Here's how the part is built. I have some questions about the finished solid (model axes, mm). A direction names the side the tool comes from. Round coordinates to 2 decimals unless told otherwise and drop trailing zeros. Write each loop counter-clockwise with the first axis right and the second up, starting at its lowest first coordinate (ties: lowest second). Pieces come first, ordered by that corner, then holes. Notation, with made-up numbers: (42.5, -10.75) - (80.5, -10.75) arc R23 ccw to (80.5, 28.25) - close; hole circle Ø11 at (66.25, 56.5). An arc over 180 degrees is marked (long way). Write item = value, one per line. Start each with the question number.
Item 1: Which directions (+Z, -Z, +X, -X, +Y, -Y) give clear straight access to the entire face, cutting with the end or side of a thin tool? Please do faces 4 (the face through (-26.398, -13, -27)), 5 (the face through (39.733, -13, 32)), 6 (the face through (39.733, -13, -32)), 7 (the face through (8, -25.4, -28)).
Item 2: If I drill on line 1 along Z through (x, y) = (-10, -7.5); line 2 along X through (y, z) = (-26, -14.5); line 3 along Z through (x, y) = (12, 2.5) (3 decimals), over which ranges is the centre line in solid material (lowest first)? Write a range as [from, to].
Item 3: If we section it at B-B (y = -20): Please give me the cut outline in (x, z) (3 decimals).
Item 4: Thinking about a two-plate mould opening in Z: for faces 1 (the face through (7, -33.02, 0)), 2 (the face through (-1, -13, 46.809)), 3 (the face through (-17.83, -12.88, -35.8)), which applies, pulls with the +Z half, pulls with the -Z half, needs draft (parallel to the pull), parting line crosses it, or undercut?
Item 5: For P1, Ø21, axis at y = -18.5, z = 25.5, coming from the -X side; P2, Ø1, axis at x = 27.5, z = 22.5, coming from the -Y side; P3, Ø20.5, axis at y = -18, z = 32, coming from the +X side, each with a flat end and sliding along its axis, tell me the tip position at first contact or that it passes through.
Item 6: If we section it at D-D (x = 29): Please give me the cut outline in (y, z) (3 decimals), and give its area (3 significant figures).
Item 7: If we section it at C-C (z = -33): Please give me the cut outline in (x, y).
Item 8: If we section it at A-A (x = 2.5): Please give me the cut outline in (y, z) (3 decimals).
```python
from build123d import *

# Parameters (mm, degrees)
F0_W      = 79.465718
F0_H      = 93.617142
F1_DEPTH  = 25.4
F3_DEPTH  = 50.292
F5_DEPTH  = 133.096
F6_W      = 68.579998
F6_H      = 34.29
F7_DEPTH  = 8.382
F7_FACE_W = 68.579998
F7_FACE_H = 34.29
F8_DEPTH  = 41.402


with BuildPart() as f1:
    # F0 (on Front) → F1 (new body)
    with BuildSketch(Plane.XZ):
        Rectangle(F0_W, F0_H)
    extrude(amount=F1_DEPTH)

    # F2 (on face) → F3 (cut)
    with BuildSketch(Plane.XZ.offset(25.4)):
        with BuildLine():
            ThreePointArc((-12.518571, 41.093569), (-17.8271, 35.919412), (-12.790714, 30.480001))
            Line((-12.790714, 30.480001), (12.246429, 30.480001))
            ThreePointArc((12.246429, 30.480001), (17.8271, 35.64718), (12.518571, 41.093569))
            Line((12.518571, 41.093569), (-12.518571, 41.093569))
        make_face()
        with BuildLine():
            ThreePointArc((12.518571, -41.093569), (17.8271, -35.64718), (12.246429, -30.480001))
            Line((12.246429, -30.480001), (-12.790714, -30.480001))
            ThreePointArc((-12.790714, -30.480001), (-17.8271, -35.919412), (-12.518571, -41.093569))
            Line((-12.518571, -41.093569), (12.518571, -41.093569))
        make_face()
    extrude(amount=-F3_DEPTH, mode=Mode.SUBTRACT)

    # F4 (on Front) → F5 (cut)
    with BuildSketch(Plane.XZ):
        Polygon((-26.397856, -36.16475), (-26.397856, 36.16475), (-42.18214, 48.441429), (-44.631425, -50.34643), align=None)
    extrude(amount=F5_DEPTH, mode=Mode.SUBTRACT)

    # F6 (on Front) → F7 (join)
    with BuildSketch(Plane.XZ):
        with Locations((7.347856, 0)):
            Rectangle(F6_W, F6_H)
    extrude(amount=-F7_DEPTH)

    # F7_face (on face) → F8 (join)
    with BuildSketch(Plane(origin=(7.347856, 8.382, 0), x_dir=(1, 0, 0), z_dir=(0, 1, 0))):
        Rectangle(F7_FACE_W, F7_FACE_H)
    extrude(amount=-F8_DEPTH)


solid = f1.part
```
Reply:
q1.face_4 = -X, +Y, -Y
q1.face_5 = +Z, +X, +Y, -Y
q1.face_6 = -Z, +X, +Y, -Y
q1.face_7 = -Z, +X, -X, -Y
q2.line_1 = [-46.81, -41.09], [-30.48, 30.48], [41.09, 46.81]
q2.line_2 = [-26.94, 41.64]
q2.line_3 = [-17.145, 17.145]
q3.outline = (-39.733, -46.809) - (39.733, -46.809) - (39.733, -17.145) - (41.638, -17.145) - (41.638, 17.145) - (39.733, 17.145) - (39.733, 46.809) - (-39.733, 46.809) - (-39.733, 46.536) - (-26.398, 36.165) - (-26.398, 17.145) - (-26.942, 17.145) - (-26.942, -17.145) - (-26.398, -17.145) - (-26.398, -36.165) - (-39.733, -46.536) - close; hole (-12.791, -30.48) arc R5.31 ccw to (-12.519, -41.094) - (12.519, -41.094) arc R5.31 ccw (long way) to (12.246, -30.48) - close; hole (-12.791, 30.48) - (12.246, 30.48) arc R5.31 ccw (long way) to (12.519, 41.094) - (-12.519, 41.094) arc R5.31 ccw to start
q4.face_1 = needs draft
q4.face_2 = pulls with the +Z half
q4.face_3 = undercut
q5.P1 = -26.94
q5.P2 = -25.4
q5.P3 = 39.73
q6.outline = (-33.02, -17.145) - (-25.4, -17.145) - (-25.4, -46.809) - (0, -46.809) - (0, -17.145) - (8.382, -17.145) - (8.382, 17.145) - (0, 17.145) - (0, 46.809) - (-25.4, 46.809) - (-25.4, 17.145) - (-33.02, 17.145) - close
q6.area = 2,930 mm2
q7.outline = (-26.4, -25.4) - (-17.04, -25.4) - (-17.04, 0) - (-26.4, 0) - close; (17.04, -25.4) - (39.73, -25.4) - (39.73, 0) - (17.04, 0) - close
q8.outline = (-33.02, -17.145) - (-25.4, -17.145) - (-25.4, -30.48) - (0, -30.48) - (0, -17.145) - (8.382, -17.145) - (8.382, 17.145) - (0, 17.145) - (0, 30.48) - (-25.4, 30.48) - (-25.4, 17.145) - (-33.02, 17.145) - close; (-25.4, -46.809) - (0, -46.809) - (0, -41.094) - (-25.4, -41.094) - close; (-25.4, 41.094) - (0, 41.094) - (0, 46.809) - (-25.4, 46.809) - close
